The figure shows three views and two pictorial views of one solid part (mm, origin at its lowest corner). Answer the questions. A direction names the side the tool comes from. Round coordinates to 2 decimals unless told otherwise and drop trailing zeros. Order: outer loops, then holes, each group sorted by start corner. A loop starts at its lowest first (then second) coordinate and runs counter-clockwise, first axis right, second up. Notation, with made-up numbers: (31, -20) - (87, -20) arc R19 ccw to (87, -14) - close; hole circle Ø1 at (49.5, -40). An arc over 180 degrees is marked (long way). Use CSV: the item, a comma, the result in double quotes.
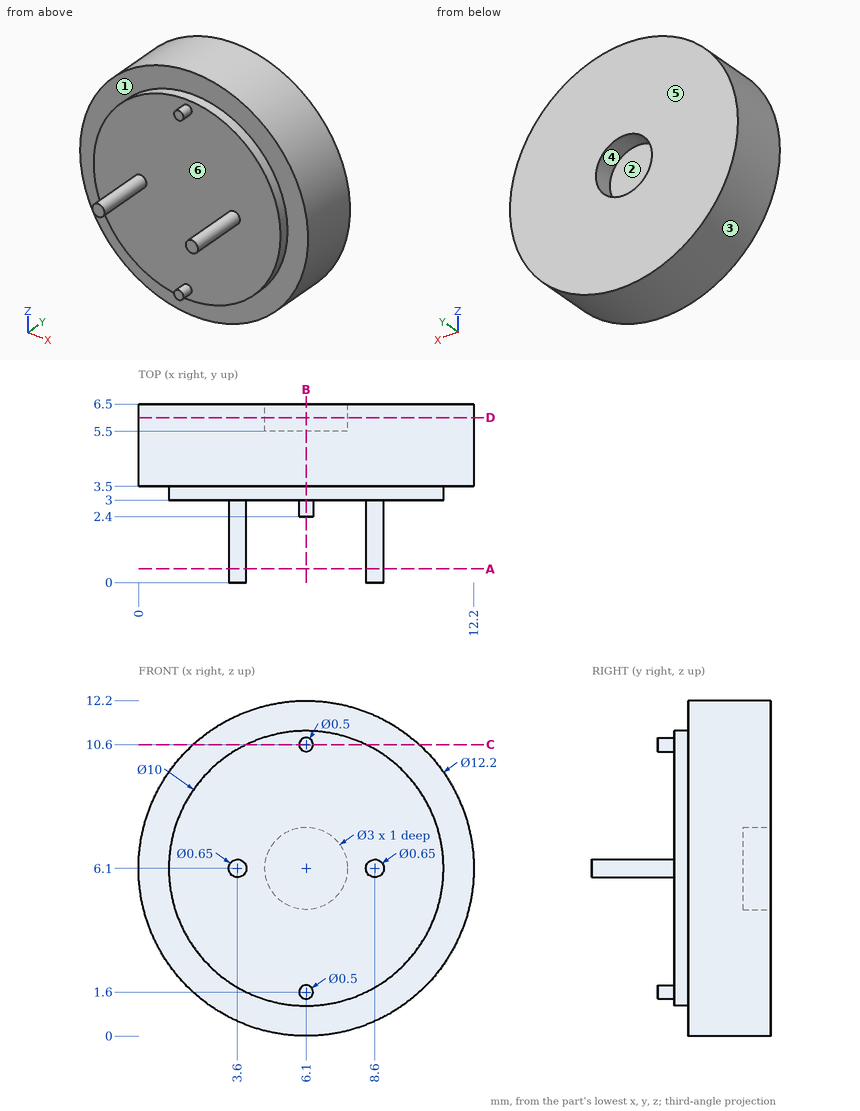
(1) Find section C-C (z = 10.6). Determine the outline of the cut face in (x, y), and give its area (3 significant figures).
Findings below:
outline,"(1.98, 3.5) - (3.92, 3.5) - (3.92, 3) - (5.85, 3) - (5.85, 2.4) - (6.35, 2.4) - (6.35, 3) - (8.28, 3) - (8.28, 3.5) - (10.22, 3.5) - (10.22, 6.5) - (1.98, 6.5) - close"
area,"27.2 mm²"
(2) Find the intervals of material crossed by L1, parallel to Z at x = 6.1, y = 6.15; L2, parallel to Y at x = 8.5, z = 4.5; L3, parallel to Y at x = 6, z = 1.5, in increasing order. Write a range as from..to.
Findings below:
L1,"z = 0..4.6, 7.6..12.2"
L2,"y = 3..6.5"
L3,"y = 2.4..6.5"
(3) Find section B-B (x = 6.1). Determine the outline of the cut face in (y, z), and give its area (3 significant figures).
Findings below:
outline,"(2.4, 1.35) - (3, 1.35) - (3, 1.1) - (3.5, 1.1) - (3.5, 0) - (6.5, 0) - (6.5, 4.6) - (5.5, 4.6) - (5.5, 7.6) - (6.5, 7.6) - (6.5, 12.2) - (3.5, 12.2) - (3.5, 11.1) - (3, 11.1) - (3, 10.85) - (2.4, 10.85) - (2.4, 10.35) - (3, 10.35) - (3, 1.85) - (2.4, 1.85) - close"
area,"39.2 mm²"
(4) Each of these flat-tipped pins is pushed along its axis until it touches: pin 1 (2 mm diameter, centred on y = 3, z = 7.5, fed in from +X); pin 2 (1 mm diameter, centred on x = 6, y = 2, fed in from +Z); pin 3 (3.5 mm diameter, centred on x = 7, z = 7, fed in from -Y); pin 4 (2 mm diameter, centred on y = 4, z = 8, fed in from +X). Where does it stop, or does it pass through?
Findings below:
pin 1,"stops at x = 12.18"
pin 2,"stops at z = 10.85"
pin 3,"stops at y = 0"
pin 4,"stops at x = 12.13"
(5) Find section D-D (y = 6). Determine the outline of the cut face in (x, z).
Findings below:
outline,"circle Ø12.2 at (6.1, 6.1); hole circle Ø3 at (6.1, 6.1)"
(6) The mould has two halves that part along Z. Classify the marked faces 1, 2 and 3: released by +Z, released by -Z, zero draft, split by the parting line, or undercut.
Findings below:
face 1,"zero draft"
face 2,"undercut"
face 3,"split by the parting line"
(7) Find section A-A (y = 0.5). Determine the outline of the cut face in (x, z) (3 decimals).
Findings below:
outline,"circle Ø0.65 at (3.6, 6.1); circle Ø0.65 at (8.6, 6.1)"
(8) For the marked faces 4, 5 and 6, determine the directions among +Z, -Z, +X, -X, +Y, -Y from which every point of the face is accessible in a straight line to the end or side of a thin tool.
Findings below:
face 4,"+Y"
face 5,"+Z, -Z, +X, -X, +Y"
face 6,"-Y"
